Geometry: see drawing. Coordinates: mm, zero at the bounding-box minimum. Round coordinates to 2 decimals unless told otherwise and drop trailing zeros. Order: outer loops, then holes, each group sorted by start corner. A loop starts at its lowest first (then second) coordinate and runs counter-clockwise, first axis right, second up. Notation, with made-up numbers: (13.25, -21.75) -> (67.25, -21.75) arc R25 cw to (67.25, 10.25) -> close; hole circle Ø10 at (58, -32.5). An arc over 180 degrees is marked (long way). Answer as CSV lines item,"result". Start each with the question number.
(1) Section query D-D (z = 73.5). Output: boundary loops of the cut face in (x, y).
(2) Section query C-C (z = 31). Output: boundary loops of the cut face in (x, y).
(3) Pull-direction query (Y, two-part tool) for the marked faces 1, 2, 3 and 4; classes: +Y half, -Y half, draft (parallel to the pull), parting line (faces both ways), or undercut.
(4) Line query: line 1 along Z through (x, y) = (11.5, 50); line 2 along Z through (x, y) = (20.25, 58.5); line 3 along Y through (x, z) = (12.5, 6). Output: solid intervals per line, ascending. Write a range as from..to.
(5) Section query B-B (z = 43). Output: boundary loops of the cut face in (x, y).
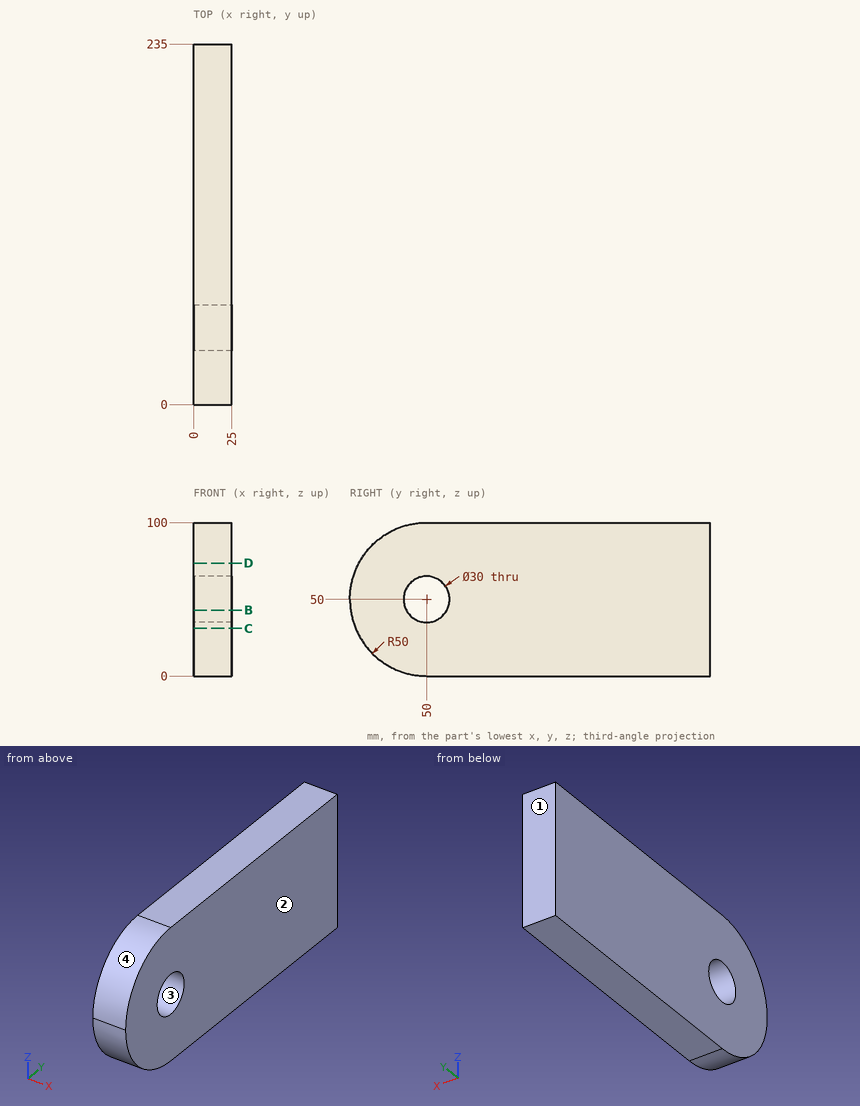
Answer block:
1,outline,"(0, 5.87) -> (25, 5.87) -> (25, 235) -> (0, 235) -> close"
2,outline,"(0, 3.75) -> (25, 3.75) -> (25, 235) -> (0, 235) -> close"
3,face 1,"+Y half"
3,face 2,"draft"
3,face 3,"undercut"
3,face 4,"-Y half"
4,line 1,"0..35, 65..100"
4,line 2,"0..37.64, 62.36..100"
4,line 3,"26.25..235"
5,outline,"(0, 0.49) -> (25, 0.49) -> (25, 36.73) -> (0, 36.73) -> close; (0, 63.27) -> (25, 63.27) -> (25, 235) -> (0, 235) -> close"
